```python
from build123d import *

# Parameters (mm, degrees)
F0_W     = 166.4
F0_H     = 116.4
F1_DEPTH = 170
F0_W_2   = 170
F0_H_2   = 120
F2_DEPTH = 170
F4_DEPTH = 1
F5_DEPTH = 5
F6_DEPTH = 170


with BuildPart() as f1:
    # F0 (on Top) → F1 (new body)
    with BuildSketch(Plane.XY):
        with Locations((6.7789069265, 121.5492137671)):
            Rectangle(F0_W, F0_H)
    extrude(amount=F1_DEPTH)


with BuildPart() as f2:
    # F0 (on Top) → F2 (new body)
    with BuildSketch(Plane.XY):
        with Locations((6.7789069265, 121.5492137671)):
            Rectangle(F0_W_2, F0_H_2)
        with Locations((6.7789069265, 121.5492137671)):
            Rectangle(F0_W, F0_H, mode=Mode.SUBTRACT)
    extrude(amount=F2_DEPTH)

    # F3: cut F1
    add(f1.part, mode=Mode.SUBTRACT)


with BuildPart() as f4:
    # F0 (on Top) → F4 (new body, symmetric)
    with BuildSketch(Plane.XY):
        with Locations((8.5789069265, -58.2)):
            Rectangle(F0_W, F0_H)
    extrude(amount=F4_DEPTH, both=True)


with BuildPart() as f5:
    # F5 (new, symmetric): a face of the model
    f5_faces = [f4.part.faces().sort_by_distance(p)[0] for p in [
        (8.5789069265, -58.2, -1),
    ]]
    extrude(f5_faces, amount=F5_DEPTH, both=True)


with BuildPart() as f4_1:
    add(f4.part)

    add(f5.part)  # F6 merges F5
    # F0 (on Top) → F6 (join)
    with BuildSketch(Plane.XY):
        with Locations((8.5789069265, -58.2)):
            Rectangle(F0_W_2, F0_H_2)
        with Locations((8.5789069265, -58.2)):
            Rectangle(F0_W, F0_H, mode=Mode.SUBTRACT)
    extrude(amount=F6_DEPTH)


solid = f4_1.part
```
Build history of the part. All positions in model axes, mm. A direction names the side the tool comes from. Coordinates: 2 decimals unless noted, no trailing zeros. Order: outer loops, then holes, each group sorted by start corner. A loop starts at its lowest first (then second) coordinate and runs counter-clockwise, first axis right, second up. Notation, with made-up numbers: M -14,79 L 37,79 A28 cw 37,99 Z; hole C 59,-23 d2. An arc over 180 degrees is marked long. One line per question, with ' | ' between items. Start each with the question number.
1. Wall check: line 1 along X through (y, z) = (-3.5, 89.5); line 2 along Y through (x, z) = (-53.5, 62); line 3 along Z through (x, y) = (-64.5, -100). Give the ranges that are in metal, low to high. Write a range as [from, to].
2. Mould opens along Y. For faces 1 (the face through (-74.621, -59, -3)), 2 (the face through (7, 0, -3)), 3 (the face through (-74.621, -59, 86)) say: +Y half, -Y half, draft (parallel to the pull), parting line (faces both ways), or undercut.
3. Cut at A-A (z = 50.5). Write the cut outline in (x, y), plus the area to 3 significant figures.
4. Cut at C-C (y = -109). Write the cut outline in (x, z), plus the area to 3 significant figures.
5. Cut at B-B (x = -0.5). Write the cut outline in (y, z).
6. Tool access for faces 4 (the face through (7, -57, -6)), 5 (the face through (91.779, -59, 86)), 6 (the face through (91.779, -59, -3)), 7 (the face through (7, -116.4, -3)): list every direction of +Z, -Z, +X, -X, +Y, -Y with a clear straight run to the whole face (end or side of a thin tool).
7. Flat gauge pins, fed straight in: P1, Ø3, axis at x = -13, z = -3, coming from the +Y side; P2, Ø12, axis at x = -38, y = -73, coming from the +Z side; P3, Ø5, axis at y = -56.5, z = -3, coming from the +X side. Where does each tip first touch, or does it go through?
The answers:
1) line 1: x = [-76.42, -74.62], [91.78, 93.58] | line 2: y = [-118.2, -116.4], [0, 1.8] | line 3: z = [-6, 4]
2) face 1: draft | face 2: +Y half | face 3: undercut
3) outline: M -76.42,-118.2 L 93.58,-118.2 L 93.58,1.8 L -76.42,1.8 Z; hole M -74.62,-116.4 L 91.78,-116.4 L 91.78,0 L -74.62,0 Z | area: 1,030 mm2
4) outline: M -76.42,0 L -74.62,0 L -74.62,-6 L 91.78,-6 L 91.78,0 L 93.58,0 L 93.58,170 L 91.78,170 L 91.78,4 L -74.62,4 L -74.62,170 L -76.42,170 Z | area: 2,280 mm2
5) outline: M -118.2,0 L -116.4,0 L -116.4,-6 L 0,-6 L 0,0 L 1.8,0 L 1.8,170 L 0,170 L 0,4 L -116.4,4 L -116.4,170 L -118.2,170 Z
6) face 4: -Z, +X, -X, +Y, -Y | face 5: +Z | face 6: -Z, +X, +Y, -Y | face 7: -Z, +X, -X, -Y
7) P1: stops at y = 0 | P2: stops at z = 4 | P3: stops at x = 91.78
